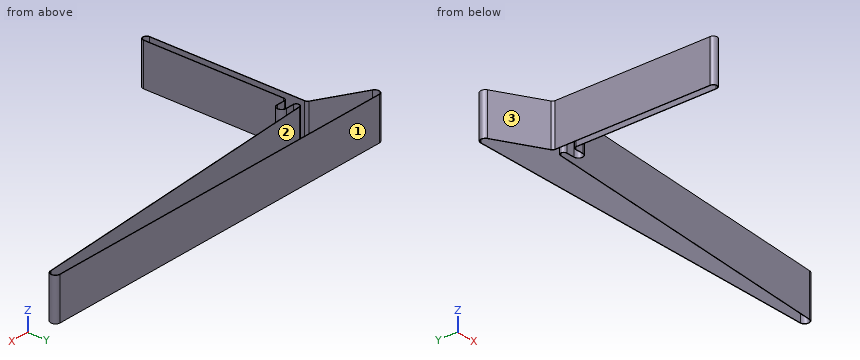
from build123d import *

# Parameters (mm, degrees)
EXTRUDE_THIN1_DEPTH = 63.5


with BuildPart() as part:
    # Sketch1 → Extrude-Thin1 (new body, symmetric)
    with BuildSketch(Plane.XY):
        with BuildLine():
            Line((-959.66739225, -104.081924367), (-934.763425273, -103.976128348))
            ThreePointArc((-934.763425273, -103.976128348), (-920.479, -118.2), (-934.763425273, -132.423871652))
            Line((-934.763425273, -132.423871652), (-959.66739225, -132.318075633))
            ThreePointArc((-959.66739225, -132.318075633), (-965.616046993, -134.759141539), (-968.084999173, -140.696276466))
            Line((-968.084999173, -140.696276466), (-968.273001128, -563.905077546))
            ThreePointArc((-968.273001128, -563.905077546), (-979.703244004, -575.329999997), (-991.132999079, -563.904589538))
            Line((-991.132999079, -563.904589538), (-991.321000676, -95.696634339))
            ThreePointArc((-991.321000676, -95.696634339), (-992.470278455, -91.463767823), (-995.600017332, -88.39086481))
            Line((-995.600017332, -88.39086481), (-1130.965637255, -12.403380928))
            ThreePointArc((-1130.965637255, -12.403380928), (-1137.764320182, 3.59836669), (-1124.003, 14.224))
            Line((-1124.003, 14.224), (0, 14.224))
            ThreePointArc((0, 14.224), (14.213745369, 0.540017203), (1.079255768, -14.182996263))
            Line((1.079255768, -14.182996263), (-960.338990006, -87.342162917))
            ThreePointArc((-960.338990006, -87.342162917), (-968.078262268, -96.036014785), (-959.66739225, -104.081924367))
        make_face()
        with BuildLine():
            Line((-959.660918114, -105.605910615), (-934.756951136, -105.500114596))
            ThreePointArc((-934.756951136, -105.500114596), (-922.003, -118.2), (-934.756951136, -130.899885404))
            Line((-934.756951136, -130.899885404), (-959.660918114, -130.794089385))
            ThreePointArc((-959.660918114, -130.794089385), (-966.691146447, -133.678985455), (-969.608999023, -140.69559946))
            Line((-969.608999023, -140.69559946), (-969.797000977, -563.90440054))
            ThreePointArc((-969.797000977, -563.90440054), (-979.70321147, -573.805999998), (-989.608999201, -563.903977599))
            Line((-989.608999201, -563.903977599), (-989.797000799, -95.696022401))
            ThreePointArc((-989.797000799, -95.696022401), (-991.155238175, -90.693543791), (-994.854020483, -87.061931139))
            Line((-994.854020483, -87.061931139), (-1130.219640407, -11.074447257))
            ThreePointArc((-1130.219640407, -11.074447257), (-1136.28989302, 3.212827402), (-1124.003, 12.7))
            Line((-1124.003, 12.7), (0, 12.7))
            ThreePointArc((0, 12.7), (12.69084408, 0.482158217), (0.963621221, -12.66338952))
            Line((0.963621221, -12.66338952), (-960.454624553, -85.822556174))
            ThreePointArc((-960.454624553, -85.822556174), (-969.601037226, -96.097108382), (-959.660918114, -105.605910615))
        make_face(mode=Mode.SUBTRACT)
    extrude(amount=EXTRUDE_THIN1_DEPTH, both=True)


solid = part.part
Verification items for the finished model (mm, model axes). Face numbers are marked on the shaded views. Give positions to 0.01 mm unless a question says otherwise; leave off trailing zeros. Write each loop counter-clockwise with the first axis right and the second up, starting at its lowest first coordinate (ties: lowest second). Pieces come first, ordered by that corner, then holes. Notation, with made-up numbers: (61, -9) - (66, -9) arc R23 cw to (66, 13) - close; hole circle Ø3 at (51, 23). An arc over 180 degrees is marked (long way). Answer as CSV lines item,"result". Start each with the question number.
1. Depth check by flat-ended pin: pin 1 (12 mm diameter, centred on y = -244, z = 8.5, fed in from -X); pin 2 (2 mm diameter, centred on y = -241, z = -16, fed in from +X); pin 3 (10 mm diameter, centred on y = -140, z = -4.5, fed in from +X). Enter the tip coordinate at first touch or a pass-through.
2. Sectioned sample at B-B (y = -47.5). Record the boundary of the cut face in (x, z), then the cut area to 3 significant figures.
3. Sectioned sample at A-A (z = -33). Record the boundary of the cut face in (x, y) (3 decimals).
4. Thickness scan on line 1 (X direction, y = -464, z = 27); line 2 (X direction, y = -304, z = 3); line 3 (Y direction, x = -1032.5, z = -13). Record the ranges inside material, lowest first.
5. Sectioned sample at C-C (x = -1009). Record the boundary of the cut face in (y, z), then the cut area to 3 significant figures.
6. Draft check along Y on the marked faces 1, 2 and 3. Enter one of: pulls with the +Y half, pulls with the -Y half, needs draft (parallel to the pull), parting line crosses it, or undercut.
Derived:
1,pin 1,"x = -991.26"
1,pin 2,"x = -968.13"
1,pin 3,"x = -965.85"
2,outline,"(-1068.44, -63.5) - (-1065.33, -63.5) - (-1065.33, 63.5) - (-1068.44, 63.5) - close; (-456.84, -63.5) - (-436.75, -63.5) - (-436.75, 63.5) - (-456.84, 63.5) - close"
2,area,"2,950 mm²"
3,outline,"(-1130.966, -12.403) - (-995.6, -88.391) arc R8.382 cw to (-991.321, -95.697) - (-991.133, -563.905) arc R11.43 ccw to (-968.273, -563.905) - (-968.085, -140.696) arc R8.382 cw to (-959.667, -132.318) - (-934.763, -132.424) arc R14.224 ccw (long way) to (-934.763, -103.976) - (-959.667, -104.082) arc R8.382 cw to (-960.339, -87.342) - (1.079, -14.183) arc R14.224 ccw to (0, 14.224) - (-1124.003, 14.224) arc R14.224 ccw to start; hole (-1130.22, -11.074) - (-994.854, -87.062) arc R9.906 cw to (-989.797, -95.696) - (-989.609, -563.904) arc R9.906 ccw to (-969.797, -563.904) - (-969.609, -140.696) arc R9.906 cw to (-959.661, -130.794) - (-934.757, -130.9) arc R12.7 ccw (long way) to (-934.757, -105.5) - (-959.661, -105.606) arc R9.906 cw to (-960.455, -85.823) - (0.964, -12.663) arc R12.7 ccw to (0, 12.7) - (-1124.003, 12.7) arc R12.7 ccw to start"
4,line 1,"-991.17 to -989.65, -969.75 to -968.23"
4,line 2,"-991.24 to -989.71, -969.68 to -968.16"
4,line 3,"-67.68 to -65.93, 12.7 to 14.22"
5,outline,"(-80.87, -63.5) - (-79.12, -63.5) - (-79.12, 63.5) - (-80.87, 63.5) - close; (12.7, -63.5) - (14.22, -63.5) - (14.22, 63.5) - (12.7, 63.5) - close"
5,area,"416 mm²"
6,face 1,"pulls with the +Y half"
6,face 2,"undercut"
6,face 3,"pulls with the -Y half"
